Check sheet for the drawn part. Datum: minimum x, y, z corner. Units: mm. Coordinates: 2 decimals unless noted, no trailing zeros. Write each loop counter-clockwise with the first axis right and the second up, starting at its lowest first coordinate (ties: lowest second). Pieces come first, ordered by that corner, then holes. Notation, with made-up numbers: (-17, 16.5) -> (-10, 16.5) arc R27 cw to (-10, 40.5) -> close; hole circle Ø7 at (-35, -15). An arc over 180 degrees is marked (long way). Answer in a Markdown table with one row per item. Add a question column.
1. Mould release check, pull along X, two halves, no side actions. Record for the marked faces 1, 2 and 3: pulls with the +X half, pulls with the -X half, needs draft (parallel to the pull), parting line crosses it, or undercut.
2. Scan lines: L1, parallel to Y at x = 10, z = 5; L2, parallel to X at y = 50, z = 5.25; L3, parallel to Y at x = 6, z = 7.5 (1 decimal). Record each from-to range of solid material in increasing order. Write a range as from..to.
3. Depth check by flat-ended pin: P1, Ø5, axis at x = 10.5, y = 40, coming from the -Z side; P2, Ø3, axis at x = 3, z = 4.5, coming from the +Y side; P3, Ø2, axis at y = 7.5, z = 7, coming from the +X side. Enter the tip coordinate at first touch or a pass-through.
4. Cross-section at C-C on x = 15.75. Record the cut outline in (y, z).
5. Cross-section at B-B on x = 6.5. Record the cut outline in (y, z).
6. Cross-section at A-A on z = 3.25. Give the number of separate pieces and of enclosed holes in the cut face, and give its area (3 significant figures).
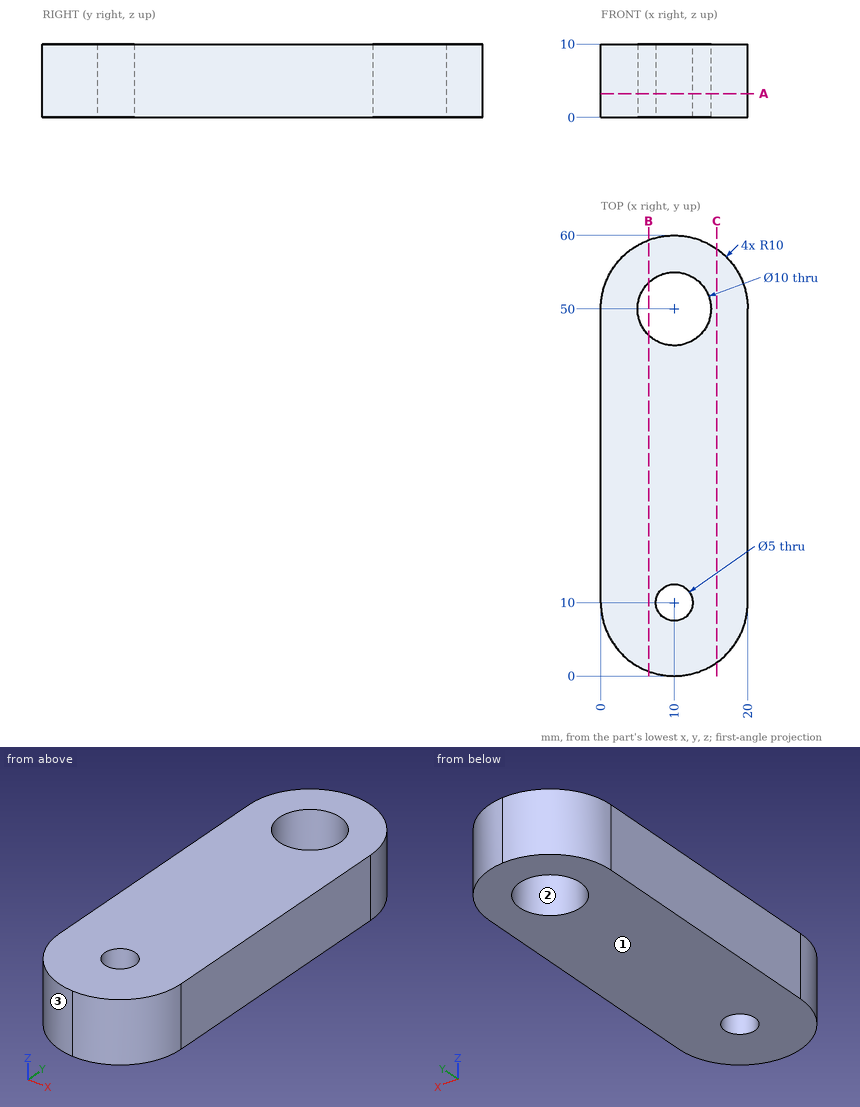
Results found:
| question | item | result |
|---|---|---|
| 1 | face 1 | needs draft |
| 1 | face 2 | undercut |
| 1 | face 3 | pulls with the -X half |
| 2 | L1 | y = 0..7.5, 12.5..45, 55..60 |
| 2 | L2 | x = 0..5, 15..20 |
| 2 | L3 | y = 0.8..47, 53..59.2 |
| 3 | P1 | stops at z = 0 |
| 3 | P2 | stops at y = 58.35 |
| 3 | P3 | stops at x = 19.89 |
| 4 | outline | (1.82, 0) -> (58.18, 0) -> (58.18, 10) -> (1.82, 10) -> close |
| 5 | outline | (0.63, 0) -> (46.43, 0) -> (46.43, 10) -> (0.63, 10) -> close; (53.57, 0) -> (59.37, 0) -> (59.37, 10) -> (53.57, 10) -> close |
| 6 | separate pieces | 1 |
| 6 | enclosed holes | 2 |
| 6 | area | 1,020 mm^2 |
